Design review of the part built by this model. Coordinates are the model's own, in mm. Give positions to 0.01 mm unless a question says otherwise; leave off trailing zeros. Order: outer loops, then holes, each group sorted by start corner. A loop starts at its lowest first (then second) coordinate and runs counter-clockwise, first axis right, second up.
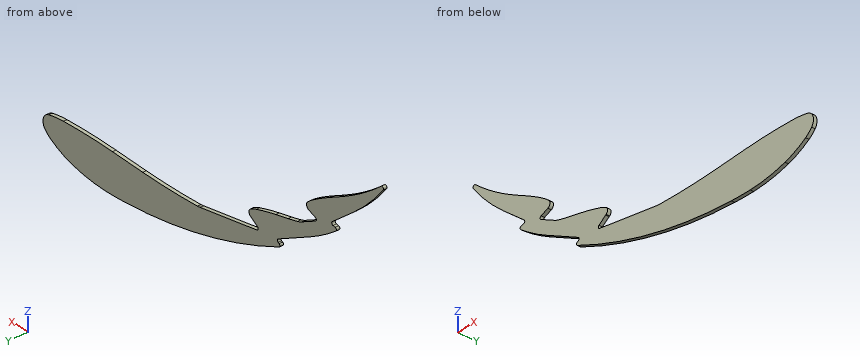
Autodesk Inventor part; units mm, degrees
ref_plane "YZ Plane" through (0, 0, 0) normal (1, 0, 0) x (0, 1, 0)
ref_plane "XZ Plane" through (0, 0, 0) normal (0, 1, 0) x (-1, 0, 0)
ref_plane "XY Plane" through (0, 0, 0) normal (0, 0, 1) x (1, 0, 0)
sketch "スケッチ1" plane through (0, 0, 0) normal (0, 1, 0) x (-1, 0, 0)
  arc A0 (317.1725, 195.8128) -> (314.2512, 198.5108) centre (315.5653, 197.0031) ccw
  arc A1 (259.4316, 139.5569) -> (317.1725, 195.8128) centre (115.0525, 345.5076) ccw
  arc A2 (250.4691, 133.6616) -> (259.4316, 139.5569) centre (155.393, 287.9636) ccw
  arc A3 (232.176, 125.5508) -> (250.4691, 133.6616) centre (211.4405, 197.0022) ccw
  arc A4 (219.6233, 123.8241) -> (232.176, 125.5508) centre (220.0183, 167.4446) ccw
  arc A5 (215.1935, 124.6186) -> (219.6233, 123.8241) centre (219.7448, 137.2497) ccw
  arc A6 (213.6042, 131.9847) -> (215.1935, 124.6186) centre (216.6995, 128.798) ccw
  arc A7 (220.1456, 137.3142) -> (213.6042, 131.9847) centre (247.3645, 97.227) ccw
  arc A8 (244.0097, 151.903) -> (220.1456, 137.3142) centre (384.6233, -104.9243) ccw
  arc A9 (244.0097, 151.903) -> (259.079, 160.1851) centre (-2315.4987, 4826.7805) ccw
  arc A10 (259.079, 160.1851) -> (286.3101, 176.9294) centre (95.2726, 457.0952) ccw
  arc A11 (286.3101, 176.9294) -> (314.2512, 198.5108) centre (118.2808, 423.3526) ccw
  arc A12 (252.3508, 120.9538) -> (250.2273, 124.316) centre (251.1064, 122.5195) ccw
  arc A13 (217.6526, 110.7016) -> (250.2273, 124.316) centre (119.1278, 392.2173) ccw
  arc A14 (187.0157, 101.5757) -> (217.6526, 110.7016) centre (105.6368, 430.7651) ccw
  arc A15 (170.3162, 97.476) -> (187.0157, 101.5757) centre (-1092.0317, 5275.5105) ccw
  arc A16 (170.3162, 97.476) -> (143.4895, 89.5609) centre (239.6668, -186.9935) ccw
  arc A17 (143.4895, 89.5609) -> (135.7916, 86.106) centre (159.4055, 43.7948) ccw
  arc A18 (135.7916, 86.106) -> (135.4203, 78.5795) centre (137.9566, 82.2268) ccw
  arc A19 (135.4203, 78.5795) -> (139.4934, 76.6657) centre (143.0857, 89.6023) ccw
  arc A20 (139.4934, 76.6657) -> (152.0654, 75.0846) centre (151.1648, 118.6976) ccw
  arc A21 (152.0654, 75.0846) -> (171.8343, 78.1844) centre (150.5294, 149.4681) ccw
  arc A22 (171.8343, 78.1844) -> (182.0173, 81.5592) centre (119.9342, 251.8363) ccw
  arc A23 (182.0173, 81.5592) -> (252.3508, 120.9538) centre (95.8618, 317.8604) ccw
  arc A24 (174.7503, 65.8482) -> (173.4237, 69.5954) centre (173.8768, 67.6474) ccw
  arc A25 (64.7746, 52.985) -> (173.4237, 69.5954) centre (11.2401, 766.801) ccw
  arc A26 (-11.9173, 50.8598) -> (64.7746, 52.985) centre (3.9096, 864.5436) ccw
  arc A27 (-53.1769, 51.7289) -> (-11.9173, 50.8598) centre (236.8377, 12839.6895) ccw
  arc A28 (-53.1769, 51.7289) -> (-120.2839, 50.0437) centre (-69.1096, -650.8128) ccw
  arc A29 (-120.2839, 50.0437) -> (-140.2753, 46.8162) centre (-111.8153, -65.9388) ccw
  arc A30 (-140.2753, 46.8162) -> (-145.8114, 29.5987) centre (-137.666, 36.4784) ccw
  arc A31 (-145.8114, 29.5987) -> (-137.5577, 22.6319) centre (-121.1943, 50.3906) ccw
  arc A32 (-137.5577, 22.6319) -> (-109.3953, 11.1574) centre (-84.3921, 112.8213) ccw
  arc A33 (-109.3953, 11.1574) -> (-61.641, 6.0637) centre (-66.7514, 184.549) ccw
  arc A34 (-61.641, 6.0637) -> (-35.9382, 7.5619) centre (-74.0904, 440.8658) ccw
  arc A35 (-35.9382, 7.5619) -> (174.7503, 65.8482) centre (-88.8837, 608.8772) ccw
  line L0 (244.0097, 125.5508) -> (251.3885, 124.4995)
  line L1 (215.1935, 124.6186) -> (228.5578, 119.8031)
  line L2 (228.5578, 119.8031) -> (203.0926, 105.9721)
  line L3 (216.5642, 97.1979) -> (170.3162, 71.9002)
  line L4 (170.3162, 71.9002) -> (174.8442, 69.3979)
  line L5 (136.0222, 78.1844) -> (149.4052, 69.4519)
  line L6 (149.4052, 69.4519) -> (64.7767, 52.9852)
  line L7 (244.0097, 125.5508) -> (276.1369, 152.3423)
  point P0 (0, 0)
extrude "押し出し1" add sketch "スケッチ1" along normal blind 4
fillet "フィレット1" radius 2 4 edges at (-228.5578, 2, 119.8031) (-149.4052, 2, 69.4519) (-244.0097, 2, 125.5508) (-170.3162, 2, 71.9002)
fillet "フィレット1" radius 30 2 edges at (-203.0926, 2, 105.9721) (-64.7767, 2, 52.9852)
properties part number "bracket2" material "木材 (オーク)"
1. For pin 1 (2 mm diameter, centred on x = 34, y = 1.5, fed in from -Z); pin 2 (1 mm diameter, centred on y = 1.5, z = 31, fed in from +X); pin 3 (1 mm diameter, centred on x = 66.5, y = 1, fed in from +Z), all flat-tipped, find the tip position at first contact; note any pin that passes through.
Recorded:
pin 1: stops at z = 7.65
pin 2: stops at x = 147.09
pin 3: stops at z = 51.91
2. For line 1 along Z through (x, y) = (-128, 2.1); line 2 along X through (y, z) = (2.85, 73.5); line 3 along Z through (x, y) = (-264, 2.95), list the stretches that pass through material, from the lowest coordinate up.
Recorded:
line 1: z = 45.54 to 65.29
line 2: x = -173.28 to -143.2
line 3: z = 142.22 to 162.95
3. Take a section at B-B (x = -105). State the section outline as (y, z) points, then the cut area to 3 significant figures.
Recorded:
outline: (0, 37.22) - (4, 37.22) - (4, 60.81) - (0, 60.81) - close
area: 94.4 mm2
4. Take a section at A-A (x = 29.5). State the section outline as (y, z) points.
Recorded:
outline: (0, 8.16) - (4, 8.16) - (4, 51.21) - (0, 51.21) - close
